For this review, use the dimensioned drawing (mm, ordinates from the lowest corner) and the shaded views. Round coordinates to 2 decimals unless told otherwise and drop trailing zeros. Order: outer loops, then holes, each group sorted by start corner. A loop starts at its lowest first (then second) coordinate and runs counter-clockwise, first axis right, second up. Notation, with made-up numbers: M 48.5,3 L 85.5,3 A16 cw 85.5,26 Z; hole C -12,40.25 d5. An arc over 180 degrees is marked long. Use a Markdown table: item, result. Add a question column.
1. Consider section A-A on z = 1.35. State the section outline as (x, y) points.
2. The part is to be moulded in two halves that separate along X. For the marked faces 1, 2 and 3, say which applies: +X half, -X half, draft (parallel to the pull), parting line (faces both ways), or undercut.
3. To check wall thickness, follow probe 1 along X at (y, z) = (5.25, 1.35) (1 decimal); probe 2 along Y at (x, z) = (4.75, 1.5) (1 decimal); probe 3 along X at (y, z) = (5.5, 1.65) (1 decimal). State the ranges of each line that lie inside material, in increasing order.
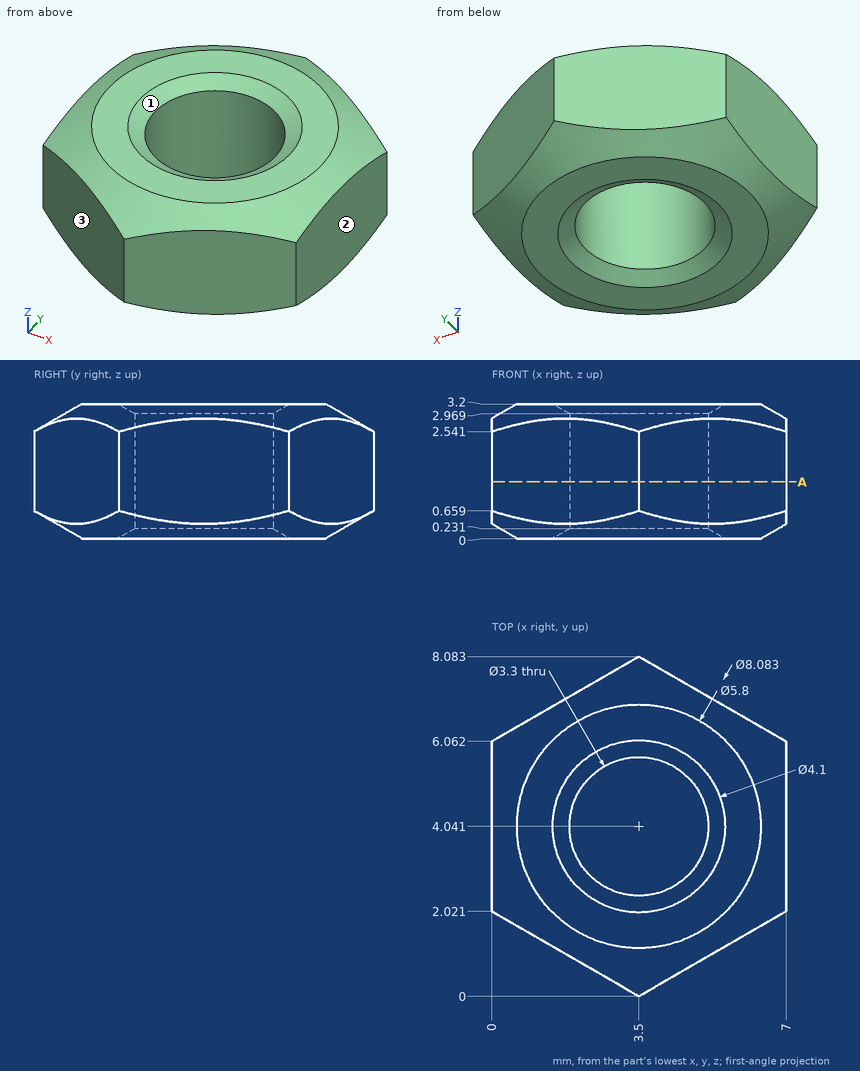
Answer block:
| question | item | result |
|---|---|---|
| 1 | outline | M 0,2.02 L 3.5,0 L 7,2.02 L 7,6.06 L 3.5,8.08 L 0,6.06 Z; hole C 3.5,4.04 d3.3 |
| 2 | face 1 | undercut |
| 2 | face 2 | +X half |
| 2 | face 3 | -X half |
| 3 | probe 1 | 0 to 2.4, 4.6 to 7 |
| 3 | probe 2 | 0.7 to 3, 5.1 to 7.4 |
| 3 | probe 3 | 0 to 2.7, 4.3 to 7 |
